```python
from build123d import *

# Parameters (mm, degrees)
SKETCH1_W                   = 254
SKETCH1_H                   = 25.4
BOSS_EXTRUDE1_DEPTH         = 6.35
SKETCH4_R                   = 4.1021
CUT_EXTRUDE4_DEPTH          = 256.345809639
F_1_4_0_25_DIAMETER_HOLE1_D = 6.35


with BuildPart() as part:
    # Sketch1 → Boss-Extrude1 (new body)
    with BuildSketch(Plane(origin=(0, 0, 0), x_dir=(1, 0, 0), z_dir=(0, 1, 0))):
        with Locations((-127, 12.7)):
            Rectangle(SKETCH1_W, SKETCH1_H)
    extrude(amount=BOSS_EXTRUDE1_DEPTH)

    # Sketch4 → Cut-Extrude4 (cut, through all)
    with BuildSketch(Plane.XZ):
        with Locations(Location((-211.4804, -12.7, 0), (0, 0, 270))):
            Circle(SKETCH4_R)
        with Locations(Location((-42.5196, -12.7, 0), (0, 0, 270))):
            Circle(SKETCH4_R)
    extrude(amount=-CUT_EXTRUDE4_DEPTH, mode=Mode.SUBTRACT)

    # 1/4 (0.25) Diameter Hole1 (through all)
    with Locations(Plane(origin=(0, 0, 0), x_dir=(-1, 0, 0), z_dir=(0, -1, 0))):
        with Locations((241.3, 12.7), (12.7, 12.7)):
            Hole(F_1_4_0_25_DIAMETER_HOLE1_D / 2)


solid = part.part
```
Work out the finished part from the listing and answer in its coordinate system (mm). Give positions to 0.01 mm unless a question says otherwise; leave off trailing zeros. Loops run counter-clockwise (first coordinate to the right, second up) from the corner with the lowest first, then second, coordinate; pieces in that order, holes last. Notation, with made-up numbers: M 59.25,6.5 L 91.25,6.5 A13 cw 91.25,13.5 Z; hole C 15,43.25 d1. An arc over 180 degrees is marked long. One line per item, written item: value. Start each with the question number.
1. Determine the mould class of faces 1 (the face through (-129, 0, -13)), 2 (the face through (-41.287, 3.131, -16.613)), 3 (the face through (-129, 3, 0)) for opening direction Z: released by +Z, released by -Z, zero draft, split by the parting line, or undercut.
2. This flat-tipped pin is pushed along its axis until it touches: P1, Ø5.5, axis at x = -241.3, z = -12.7, coming from the +Y side. Where does it stop, or does it pass through?
3. Find section B-B (x = -12.7). Give the vertices of the cut face in (y, z) (3 decimals), and give its area (3 significant figures).
4. Find section A-A (z = -12.7). State how many separate pieces and enclosed holes the cut face has, and give its area (3 significant figures).
5. Find section C-C (y = 2.75). Give the vertices of the cut face in (x, z) (3 decimals), and give its area (3 significant figures).
6. Find the intervals of material crossed by probe 1 along X at (y, z) = (2.5, -12.7) (1 decimal); probe 2 along Z at (x, y) = (-241.3, 2.25) (3 decimals); probe 3 along X at (y, z) = (6, -10.5), in increasing order.
Reported:
1. face 1: zero draft
1. face 2: undercut
1. face 3: released by +Z
2. P1: passes through
3. outline: M 0,-25.4 L 6.35,-25.4 L 6.35,-15.875 L 0,-15.875 Z; M 0,-9.525 L 6.35,-9.525 L 6.35,0 L 0,0 Z
3. area: 121 mm²
4. separate pieces: 5
4. enclosed holes: 0
4. area: 1,430 mm²
5. outline: M -254,-25.4 L 0,-25.4 L 0,0 L -254,0 Z; hole C -241.3,-12.7 d6.35; hole C -211.48,-12.7 d8.204; hole C -42.52,-12.7 d8.204; hole C -12.7,-12.7 d6.35
5. area: 6,280 mm²
6. probe 1: x = -254 to -244.5, -238.1 to -215.6, -207.4 to -46.6, -38.4 to -15.9, -9.5 to 0
6. probe 2: z = -25.4 to -15.875, -9.525 to 0
6. probe 3: x = -254 to -243.59, -239.01 to -214.94, -208.02 to -45.98, -39.06 to -14.99, -10.41 to 0
